Work out the finished part from the listing and answer in its coordinate system (mm). Face numbers are marked on the shaded views. A direction names the side the tool comes from. Give positions to 0.01 mm unless a question says otherwise; leave off trailing zeros. Loops run counter-clockwise (first coordinate to the right, second up) from the corner with the lowest first, then second, coordinate; pieces in that order, holes last. Notation, with made-up numbers: (33, 82) - (76, 82) arc R36 ccw to (76, 119) - close; hole circle Ø6 at (-28.5, 64.5). An arc over 180 degrees is marked (long way). One line per item, written item: value.
from build123d import *

# Parameters (mm, degrees)
F0_R     = 10
F1_DEPTH = 50
F3_DEPTH = 20
F5_DEPTH = 50
F6_R     = 9.99999


# Not quite as in the source:
# - a fillet or chamfer is up to 0.001 mm smaller than in the source, because OpenCascade refuses the exact size


with BuildPart() as f1:
    # F0 (on Top) → F1 (new body)
    with BuildSketch(Plane.XY):
        Circle(F0_R)
    extrude(amount=F1_DEPTH)

    # F2 (on face) → F3 (join)
    with BuildSketch(Plane.XY.offset(50)):
        with BuildLine():
            ThreePointArc((10, 0), (0, -10), (-10, 0))
            Line((-10, 0), (-10, -70))
            Line((-10, -70), (10, -70))
            Line((10, -70), (10, 0))
        make_face()
    extrude(amount=-F3_DEPTH)

    # F4 (on face) → F5 (join)
    with BuildSketch(Plane.XY.offset(50)):
        with BuildLine():
            Line((-10, -35), (-10, -70))
            ThreePointArc((-10, -70), (0, -60), (10, -70))
            Line((10, -70), (10, -35))
            Line((10, -35), (-10, -35))
        make_face()
        with BuildLine():
            ThreePointArc((10, -70), (0, -60), (-10, -70))
            Line((-10, -70), (10, -70))
        make_face()
        with BuildLine():
            Line((10, -70), (-10, -70))
            ThreePointArc((-10, -70), (0, -80), (10, -70))
        make_face()
    extrude(amount=-F5_DEPTH)

    # F6 (radius 10 in the source; OpenCascade refuses exactly that, so slightly less here)
    f6_edges = [f1.edges().sort_by_distance(p)[0] for p in [
        (10, -35, 15),
        (-10, -35, 15),
    ]]
    fillet(f6_edges, radius=F6_R)


solid = f1.part
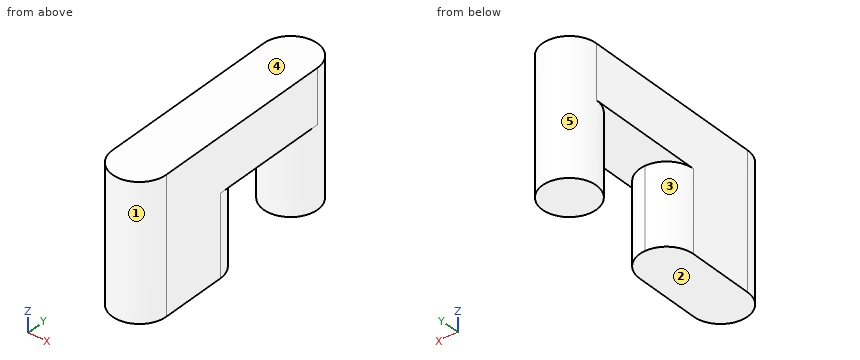
1. For the marked faces 4 and 5, determine the directions among +Z, -Z, +X, -X, +Y, -Y from which every point of the face is accessible in a straight line to the end or side of a thin tool.
Output:
face 4: +Z, +X, -X, +Y, -Y
face 5: -Z
2. The mould has two halves that part along Y. Classify the marked faces 1, 2 and 3: released by +Y, released by -Y, zero draft, split by the parting line, or undercut.
Output:
face 1: released by -Y
face 2: zero draft
face 3: undercut
3. Section A-A (x = 6) is taken. Write down the section's boundary in (y, z), and give its area (3 significant figures).
Output:
outline: (-78, 0) - (-37, 0) - (-37, 30) - (-8, 30) - (-8, 0) - (8, 0) - (8, 50) - (-78, 50) - close
area: 3,430 mm²
4. Flat-ended cylindrical pins translate along their axes: pin 1 Ø2 at (x, z) = (6.5, 7.5) entering from +Y; pin 2 Ø3 at (x, z) = (4, 43.5) entering from -Y; pin 3 Ø1.5 at (x, y) = (6.5, -33) entering from -Z. Find the tip coordinate at first contact, or state that the pin passes through.
Output:
pin 1: stops at y = 8.35
pin 2: stops at y = -79.68
pin 3: stops at z = 30
5. Find the intervals of material crossed by line 1 along Z through (x, y) = (0.5, -23); line 2 along Y through (x, z) = (7, 6.5); line 3 along Y through (x, z) = (6.25, 24), in increasing order.
Output:
line 1: z = 30 to 50
line 2: y = -77.14 to -37.86, -7.14 to 7.14
line 3: y = -77.81 to -37.19, -7.81 to 7.81
6. Section B-B (y = -9) is taken. Write down the section's boundary in (x, z), and give its area (3 significant figures).
Output:
outline: (-10, 30) - (-4.36, 30) - (-4.36, 0) - (4.36, 0) - (4.36, 30) - (10, 30) - (10, 50) - (-10, 50) - close
area: 662 mm²
